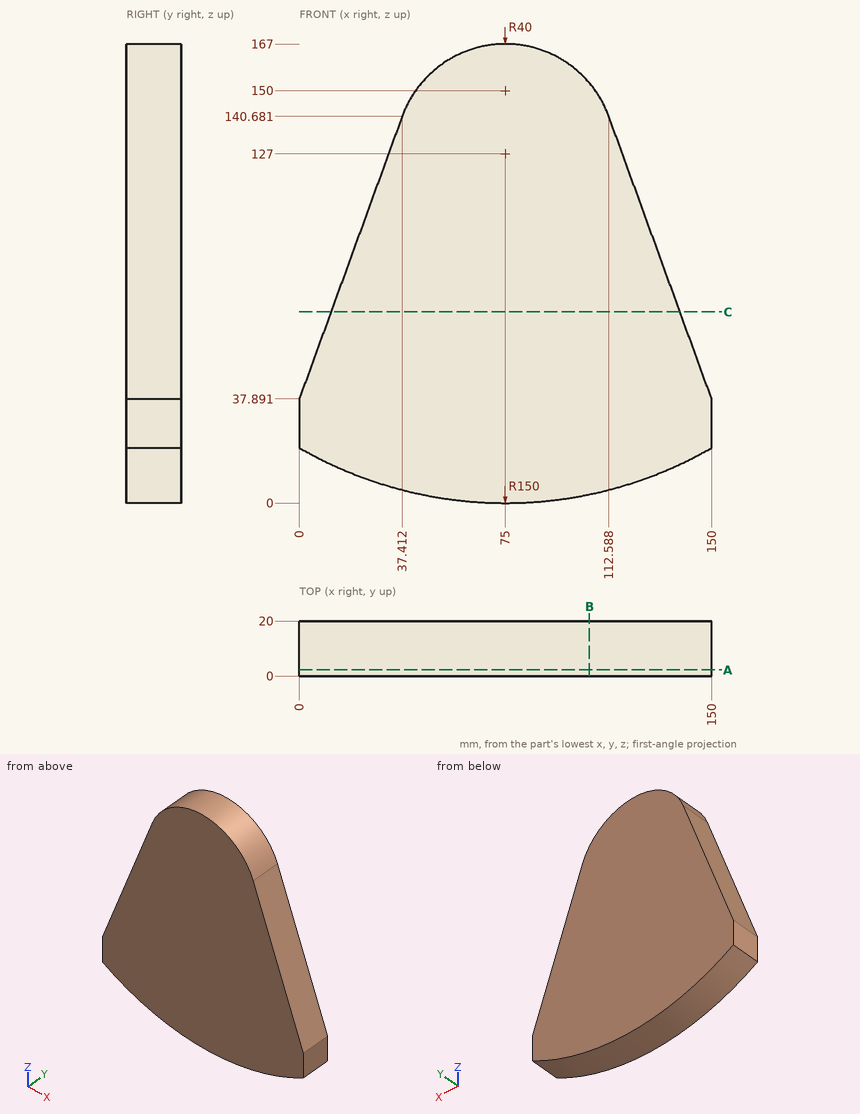
For this review, use the dimensioned drawing (mm, ordinates from the lowest corner) and the shaded views. Round coordinates to 2 decimals unless told otherwise and drop trailing zeros. Write each loop counter-clockwise with the first axis right and the second up, starting at its lowest first coordinate (ties: lowest second). Pieces come first, ordered by that corner, then holes. Notation, with made-up numbers: (25, 69) -> (55, 69) arc R25 ccw to (55, 104) -> close; hole circle Ø2 at (20, -20.5). An arc over 180 degrees is marked (long way). Answer in a Markdown table with one row per item.
Q1. Take a section at C-C, the plane z = 69.5. State the section outline as (x, y) points (1 decimal), then the cut area to 3 significant figures.
The answers:
| item | result |
|---|---|
| outline | (11.5, 0) -> (138.5, 0) -> (138.5, 20) -> (11.5, 20) -> close |
| area | 2,540 mm² |
Q2. Take a section at A-A, the plane y = 2.25. State the section outline as (x, z) points, then the cut area to 3 significant figures.
The answers:
| item | result |
|---|---|
| outline | (0, 20.1) arc R150 ccw to (150, 20.1) -> (150, 37.89) -> (112.59, 140.68) arc R40 ccw to (37.41, 140.68) -> (0, 37.89) -> close |
| area | 17,700 mm² |
Q3. Clearance check with flat-ended pins moving along their axes: pin 1 Ø10 at (y, z) = (15.5, 130) entering from +X (1 decimal); pin 2 Ø10 at (y, z) = (5, 65) entering from -X; pin 3 Ø2 at (x, y) = (128, 4) entering from -Z. State where each tip first meets the part, or that it passes through.
The answers:
| item | result |
|---|---|
| pin 1 | x = 118.3 |
| pin 2 | x = 8.05 |
| pin 3 | z = 9.3 |
Q4. To check wall thickness, follow L1, parallel to X at y = 8, z = 130 (1 decimal); L2, parallel to X at y = 18.25, z = 40.5; L3, parallel to Z at x = 93.5, y = 13.25 (1 decimal). State the ranges of each line that lie inside material, in increasing order. Write a range as [from, to].
The answers:
| item | result |
|---|---|
| L1 | [33.5, 116.5] |
| L2 | [0.95, 149.05] |
| L3 | [1.1, 162.5] |
Q5. Take a section at B-B, the plane x = 105.5. State the section outline as (y, z) points.
The answers:
| item | result |
|---|---|
| outline | (0, 3.13) -> (20, 3.13) -> (20, 152.88) -> (0, 152.88) -> close |
